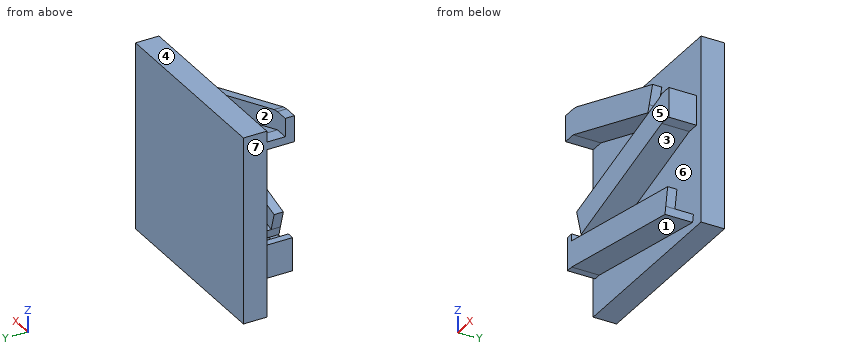
```python
from build123d import *

# Parameters (mm, degrees)
F0_W      = 203.2
F0_H      = 203.2
F1_DEPTH  = 12.7
F3_DEPTH  = 30
F4_W      = 14.6268990993
F4_H      = 10
F5_DEPTH  = 20
F6_W      = 150.9801479243
F6_H      = 10
F7_DEPTH  = 20
F9_DEPTH  = 10
F10_W     = 160.9058431263
F10_H     = 10
F11_DEPTH = 20
F12_W     = 180.2359047158
F12_H     = 10
F13_DEPTH = 20
F15_DEPTH = 10
F17_DEPTH = 10


with BuildPart() as f1:
    # F0 (on Front) → F1 (new body, symmetric)
    with BuildSketch(Plane.XZ):
        Rectangle(F0_W, F0_H)
    extrude(amount=F1_DEPTH, both=True)

    # F2 (on face) → F3 (join)
    with BuildSketch(Plane.XZ.offset(12.7)):
        Polygon((-86.9731009007, 89.6006897092), (-101.6, 89.6006897092), (-101.6, 81.2605177762), (-86.9731009007, 81.2605177762), (53.4253248086, 33.5147284107), (55.9675842524, 40.99034518), align=None)
        Polygon((92.9285819118, 40.99034518), (79.5278856938, 40.99034518), (79.5278856938, 19.016228551), (79.5278856938, 8.5395236786), (92.9285819118, 8.5395236786), align=None)
        Polygon((79.5278856938, 8.5395236786), (79.5278856938, 19.016228551), (-75.126208961, -25.4), (-72.3465969379, -35.0784079816), align=None)
        Polygon((-90.126208961, -25.4), (-98.0089604855, -25.4), (-98.0089604855, -61.6170221653), (-90.126208961, -61.6170221653), (-90.126208961, -53.2994725252), align=None)
        Polygon((-90.126208961, -53.2994725252), (-90.126208961, -61.6170221653), (85.6593027711, -93.9363369431), (87.1385357673, -85.8907539536), align=None)
    extrude(amount=F3_DEPTH)

    # F4 (on face) → F5 (join)
    with BuildSketch(Plane.XY.offset(89.6006897092)):
        with Locations((-94.2865504503, -37.7)):
            Rectangle(F4_W, F4_H)
    extrude(amount=F5_DEPTH)

    # F6 (on face) → F7 (join)
    with BuildSketch(Plane(origin=(18.2964041178, 0, 53.8013166903), x_dir=(0.9467515241, 0, -0.3219651404), z_dir=(0.3219651404, 0, 0.9467515241))):
        with Locations((-35.7001405146, -37.7)):
            Rectangle(F6_W, F6_H)
    extrude(amount=F7_DEPTH)

    # F8 (on face) → F9 (join)
    with BuildSketch(Plane.XZ.offset(42.7)):
        Polygon((-86.9731009007, 109.6006897092), (-86.9731009007, 89.6006897092), (-80.533798092, 108.5357201908), align=None)
    extrude(amount=-F9_DEPTH)

    # F10 (on face) → F11 (join)
    with BuildSketch(Plane(origin=(1.0145486096, 0, -3.532584864), x_dir=(0.9611465417, 0, 0.2760386303), z_dir=(-0.2760386303, 0, 0.9611465417))):
        with Locations((1.234244421, -37.7)):
            Rectangle(F10_W, F10_H)
    extrude(amount=F11_DEPTH)

    # F12 (on face) → F13 (join)
    with BuildSketch(Plane(origin=(-12.4259747266, 0, -67.5851682222), x_dir=(0.9835151604, 0, -0.1808256878), z_dir=(0.1808256878, 0, 0.9835151604))):
        with Locations((11.1153732758, -37.7)):
            Rectangle(F12_W, F12_H)
    extrude(amount=F13_DEPTH)

    # F14 (on face) → F15 (join)
    with BuildSketch(Plane.XZ.offset(42.7)):
        Polygon((74.0071130869, 38.2391593843), (79.5278856938, 19.016228551), (79.5278856938, 40.99034518), align=None)
    extrude(amount=-F15_DEPTH)

    # F16 (on face) → F17 (join)
    with BuildSketch(Plane.XZ.offset(42.7)):
        Polygon((-90.126208961, -32.9642496368), (-90.126208961, -53.2994725252), (-86.5096952059, -33.6291693182), align=None)
    extrude(amount=-F17_DEPTH)


solid = f1.part
```
The listing builds one solid part. Answer for the finished solid, in the listing's coordinates (mm). Face numbers are marked on the shaded views. A direction names the side the tool comes from. Give positions to 0.01 mm unless a question says otherwise; leave off trailing zeros. Order: outer loops, then holes, each group sorted by start corner. A loop starts at its lowest first (then second) coordinate and runs counter-clockwise, first axis right, second up. Notation, with made-up numbers: (16, 10) -> (35, 10) arc R16 ccw to (35, 17) -> close; hole circle Ø1 at (-17, 27). An arc over 180 degrees is marked (long way). Answer as a JSON object with one key per item and string values. Group by question number.
Item 1: The part is cut by section B-B on z = 26. Write down the section's boundary in (x, y).
Item 2: Determine the mould class of the marked faces 5, 6 and 7 for opening direction Y: pulls with the +Y half, pulls with the -Y half, needs draft (parallel to the pull), parting line crosses it, or undercut.
Item 3: The part is cut by section A-A on y = -19.5. Write down the section's boundary in (x, z), and give its area (3 significant figures).
Item 4: Consider L1, parallel to Y at x = 75.5, z = -78; L2, parallel to Z at x = -40.5, y = -25; L3, parallel to Z at x = -42, y = -1.5. Determine where each line is inside the solid, lowest interval first. Write a range as from..to.
Item 5: The part is cut by section C-C on x = -15. Write down the section's boundary in (y, z).
Item 6: The part is cut by section D-D on y = -8. Write down the section's boundary in (x, z).
Item 7: A tool of negligible diameter and unlimited length cuts with its end or side. For the marked faces 1, 2, 3 and 4, from which of +Z, -Z, +X, -X, +Y, -Y can it reach the whole face along a straight path? Write none if from no direction.
Item 8: Flat-ended cylindrical pins translate along their axes: pin 1 (7.5 mm diameter, centred on x = -96, y = -27.5, fed in from +Z); pin 2 (6.5 mm diameter, centred on x = 88, y = -27.5, fed in from +Z); pin 3 (11.5 mm diameter, centred on x = -94.5, y = -23.5, fed in from -Z). Find the tip coordinate at first contact, or state that the pin passes through.
Result set:
{
 "1": {"outline": "(-101.6, -12.7) -> (79.53, -12.7) -> (79.53, -32.7) -> (31.39, -32.7) -> (31.39, -42.7) -> (92.93, -42.7) -> (92.93, -12.7) -> (101.6, -12.7) -> (101.6, 12.7) -> (-101.6, 12.7) -> close"},
 "2": {"face 5": "pulls with the -Y half", "face 6": "undercut", "face 7": "needs draft"},
 "3": {"outline": "(-101.6, 81.26) -> (-86.97, 81.26) -> (53.43, 33.51) -> (55.97, 40.99) -> (-86.97, 89.6) -> (-101.6, 89.6) -> close; (-98.01, -61.62) -> (-90.13, -61.62) -> (85.66, -93.94) -> (87.14, -85.89) -> (-90.13, -53.3) -> (-90.13, -25.4) -> (-98.01, -25.4) -> close; (-75.13, -25.4) -> (-72.35, -35.08) -> (79.53, 8.54) -> (92.93, 8.54) -> (92.93, 40.99) -> (79.53, 40.99) -> (79.53, 19.02) -> close", "area": "5,100 mm²"},
 "4": {"L1": "-42.7..-32.7, -12.7..12.7", "L2": "-70.74..-62.42, -25.93..-15.46, 65.46..73.8", "L3": "-101.6..101.6"},
 "5": {"outline": "(-42.7, -75.43) -> (-12.7, -75.43) -> (-12.7, -101.6) -> (12.7, -101.6) -> (12.7, 101.6) -> (-12.7, 101.6) -> (-12.7, 65.12) -> (-32.7, 65.12) -> (-32.7, 86.25) -> (-42.7, 86.25) -> (-42.7, 56.78) -> (-12.7, 56.78) -> (-12.7, -8.13) -> (-32.7, -8.13) -> (-32.7, 12.68) -> (-42.7, 12.68) -> (-42.7, -18.61) -> (-12.7, -18.61) -> (-12.7, -67.11) -> (-32.7, -67.11) -> (-32.7, -46.78) -> (-42.7, -46.78) -> close"},
 "6": {"outline": "(-101.6, -101.6) -> (101.6, -101.6) -> (101.6, 101.6) -> (-101.6, 101.6) -> close"},
 "7": {"face 1": "-Z, -X, -Y", "face 2": "+Z, +X", "face 3": "+X, -Y", "face 4": "+Z, +X, -X, +Y"},
 "8": {"pin 1": "z = 89.6", "pin 2": "z = 40.99", "pin 3": "z = -61.87"}
}
